from build123d import *

# Parameters (mm, degrees)
SKETCH1_W                 = 17.526
SKETCH1_H                 = 19.05
BOSS_EXTRUDE1_DEPTH       = 6.604
M3X0_5_TAPPED_HOLE1_D     = 2.5
M3X0_5_TAPPED_HOLE1_DEPTH = 7.493
M3X0_5_TAPPED_HOLE1_TIP   = 0.751075774
M3X0_5_TAPPED_HOLE2_D     = 2.5
M3X0_5_TAPPED_HOLE2_DEPTH = 7.493
M3X0_5_TAPPED_HOLE2_TIP   = 0.751075774


with BuildPart() as part:
    # Sketch1 → Boss-Extrude1 (new body)
    with BuildSketch(Plane.XY):
        Rectangle(SKETCH1_W, SKETCH1_H)
    extrude(amount=BOSS_EXTRUDE1_DEPTH)

    # M3x0.5 Tapped Hole1
    with Locations(Plane(origin=(0, 9.525, 0), x_dir=(1, 0, 0), z_dir=(0, 1, 0))):
        with Locations((0, -3.302)):
            Hole(M3X0_5_TAPPED_HOLE1_D / 2, depth=M3X0_5_TAPPED_HOLE1_DEPTH)
            with Locations((0, 0, -(M3X0_5_TAPPED_HOLE1_DEPTH + M3X0_5_TAPPED_HOLE1_TIP / 2))):  # 118° drill point
                Cone(0, M3X0_5_TAPPED_HOLE1_D / 2, M3X0_5_TAPPED_HOLE1_TIP, mode=Mode.SUBTRACT)

    # M3x0.5 Tapped Hole2
    with Locations(Plane(origin=(0, -9.525, 0), x_dir=(-1, 0, 0), z_dir=(0, -1, 0))):
        with Locations((0, -3.302)):
            Hole(M3X0_5_TAPPED_HOLE2_D / 2, depth=M3X0_5_TAPPED_HOLE2_DEPTH)
            with Locations((0, 0, -(M3X0_5_TAPPED_HOLE2_DEPTH + M3X0_5_TAPPED_HOLE2_TIP / 2))):  # 118° drill point
                Cone(0, M3X0_5_TAPPED_HOLE2_D / 2, M3X0_5_TAPPED_HOLE2_TIP, mode=Mode.SUBTRACT)


solid = part.part
Geometry: final body of the model. Coordinates: model frame, mm. A direction names the side the tool comes from. Coordinates: 2 decimals unless noted, no trailing zeros. Order: outer loops, then holes, each group sorted by start corner. A loop starts at its lowest first (then second) coordinate and runs counter-clockwise, first axis right, second up.
(1) Access query for faces 1 (the face through (-8.763, 0, 3)), 2 (the face through (-0.163, -5.726, 2.063)). Directions: +Z, -Z, +X, -X, +Y, -Y. A direction counts if a zero-diameter tool reaches every point of the face in a straight line with its end or side. Return the directions, or none.
(2) First-contact query: pin 1 (1 mm diameter, centred on x = -0.5, z = 4, fed in from +Y) (3 decimals). Flat tip, straight axial feed; report the tip coordinate or a pass-through.
(3) Material intervals for probe 1 along Z at (x, y) = (0, 7); probe 2 along X at (y, z) = (-7.75, 2.75); probe 3 along X at (y, z) = (-8.5, 3.5), sorted ascending.
(4) Section query A-A (y = -4.25). Return the cut outline in (x, z), plus the area to 3 significant figures.
(5) Draft query along Z for faces 3 (the face through (0.163, 5.726, 2.063)), 4 (the face through (-0.1, -9.525, 1.8)), 5 (the face through (0, 0, 6.604)). Return one class per face: pulls with the +Z half, pulls with the -Z half, needs draft (parallel to the pull), parting line crosses it, or undercut.
Solution:
1. face 1: +Z, -Z, -X, +Y, -Y
1. face 2: -Y
2. pin 1: stops at y = 9.525
3. probe 1: z = 0 to 2.05, 4.55 to 6.6
3. probe 2: x = -8.76 to -1.12, 1.12 to 8.76
3. probe 3: x = -8.76 to -1.23, 1.23 to 8.76
4. outline: (-8.76, 0) - (8.76, 0) - (8.76, 6.6) - (-8.76, 6.6) - close; hole circle Ø2.5 at (0, 3.3)
4. area: 111 mm2
5. face 3: undercut
5. face 4: needs draft
5. face 5: pulls with the +Z half
